Geometry: final body of the model. Coordinates: model frame, mm. A direction names the side the tool comes from. Give positions to 0.01 mm unless a question says otherwise; leave off trailing zeros. Write each loop counter-clockwise with the first axis right and the second up, starting at its lowest first coordinate (ties: lowest second). Pieces come first, ordered by that corner, then holes.
```python
from build123d import *

# Parameters (mm, degrees)
SKETCH1_R           = 31.5
BOSS_EXTRUDE4_DEPTH = 10
SKETCH3_R           = 3
CUT_EXTRUDE2_DEPTH  = 10
SKETCH4_R           = 5
CUT_EXTRUDE3_DEPTH  = 5
SKETCH5_R           = 2.5
BOSS_EXTRUDE5_DEPTH = 13


with BuildPart() as part:
    # Sketch1 → Boss-Extrude4 (new body)
    with BuildSketch(Plane(origin=(0, 0, 0), x_dir=(1, 0, 0), z_dir=(0, 1, 0))):
        with Locations(Location((0, 0, 0), (0, 0, 270))):
            Circle(SKETCH1_R)
    extrude(amount=BOSS_EXTRUDE4_DEPTH)

    # Sketch3 → Cut-Extrude2 (cut)
    with BuildSketch(Plane(origin=(0, 0, 0), x_dir=(1, 0, 0), z_dir=(0, 1, 0))):
        with Locations(Location((0, 25, 0), (0, 0, 270))):
            Circle(SKETCH3_R)
        with Locations(Location((25, 0, 0), (0, 0, 270))):
            Circle(SKETCH3_R)
        with Locations(Location((0, -25, 0), (0, 0, 270))):
            Circle(SKETCH3_R)
        with Locations(Location((-25, 0, 0), (0, 0, 270))):
            Circle(SKETCH3_R)
    extrude(amount=CUT_EXTRUDE2_DEPTH, mode=Mode.SUBTRACT)

    # Sketch4 → Cut-Extrude3 (cut)
    with BuildSketch(Plane(origin=(0, 0, 0), x_dir=(1, 0, 0), z_dir=(0, 1, 0))):
        with Locations(Location((0, 25, 0), (0, 0, 270))):
            Circle(SKETCH4_R)
        with Locations(Location((25, 0, 0), (0, 0, 270))):
            Circle(SKETCH4_R)
        with Locations(Location((0, -25, 0), (0, 0, 270))):
            Circle(SKETCH4_R)
        with Locations(Location((-25, 0, 0), (0, 0, 270))):
            Circle(SKETCH4_R)
    extrude(amount=CUT_EXTRUDE3_DEPTH, mode=Mode.SUBTRACT)

    # Sketch5 → Boss-Extrude5 (add)
    with BuildSketch(Plane(origin=(0, 0, 0), x_dir=(1, 0, 0), z_dir=(0, 1, 0))):
        with BuildLine():
            Line((-40.658639918, -26.516504294), (26.516504294, 40.658639918))
            ThreePointArc((26.516504294, 40.658639918), (40.658639918, 40.658639918), (40.658639918, 26.516504294))
            Line((40.658639918, 26.516504294), (-26.516504294, -40.658639918))
            ThreePointArc((-26.516504294, -40.658639918), (-40.658639918, -40.658639918), (-40.658639918, -26.516504294))
        make_face()
        with Locations(Location((-33.587572106, -33.587572106, 0), (0, 0, 270))):
            Circle(SKETCH5_R, mode=Mode.SUBTRACT)
        with Locations(Location((33.587572106, 33.587572106, 0), (0, 0, 270))):
            Circle(SKETCH5_R, mode=Mode.SUBTRACT)
    extrude(amount=-BOSS_EXTRUDE5_DEPTH)


solid = part.part
```
Item 1: Section A-A, the plane x = 0. Return the cut outline in (y, z).
Found:
outline: (-13, -14.14) - (0, -14.14) - (0, -20) - (5, -20) - (5, -22) - (10, -22) - (10, 22) - (5, 22) - (5, 20) - (0, 20) - (0, 14.14) - (-13, 14.14) - close; (0, -31.5) - (10, -31.5) - (10, -28) - (5, -28) - (5, -30) - (0, -30) - close; (0, 30) - (5, 30) - (5, 28) - (10, 28) - (10, 31.5) - (0, 31.5) - close
Item 2: Section B-B, the plane z = 24. Return the cut outline in (x, y).
Found:
outline: (-38.14, -13) - (-9.86, -13) - (-9.86, 0) - (-4.9, 0) - (-4.9, 5) - (-2.83, 5) - (-2.83, 10) - (-20.4, 10) - (-20.4, 0) - (-38.14, 0) - close; (2.83, 5) - (4.9, 5) - (4.9, 0) - (20.4, 0) - (20.4, 10) - (2.83, 10) - close
Item 3: Reachability of faces 5 (the face through (-29.88, 2.46, -1.08)), 6 (the face through (14, 0, 13)), 7 (the face through (-13, 0, -14)), 8 (the face through (40.501, -6.409, -40.812)), 9 (the face through (31.232, 4.93, -4.101)) from +Z, -Z, +X, -X, +Y, -Y: full face, straight path, thin tool, end or side. Return the list, or none.
Found:
face 5: -Y
face 6: +Z, +X, -Y
face 7: -Z, -X, -Y
face 8: +Y, -Y
face 9: +Y
Item 4: Line query: L1, parallel to X at y = 7.5, z = 0; L2, parallel to X at y = 3, z = 0. Output: solid intervals per line, ascending.
Found:
L1: x = -31.5 to -28, -22 to 22, 28 to 31.5
L2: x = -31.5 to -30, -20 to 20, 30 to 31.5
Item 5: Pin query (flat end, axial travel): pin 1 Ø2 at (x, y) = (-24, -4) entering from -Z; pin 2 Ø16 at (x, z) = (0, -25) entering from -Y; pin 3 Ø8 at (x, z) = (26, 2) entering from -Y; pin 4 Ø4 at (y, z) = (0.5, 20) entering from +X. Return the tip coordinate at first contact, or that it passes through.
Found:
pin 1: stops at z = 8.86
pin 2: stops at y = -13
pin 3: stops at y = 0
pin 4: stops at x = 25.85
Item 6: Section C-C, the plane x = 25. Return the cut outline in (y, z).
Found:
outline: (-13, -39.14) - (0, -39.14) - (0, -19.16) - (10, -19.16) - (10, -3) - (5, -3) - (5, -5) - (0, -5) - (0, -10.86) - (-13, -10.86) - close; (0, 5) - (5, 5) - (5, 3) - (10, 3) - (10, 19.16) - (0, 19.16) - close
Item 7: Section D-D, the plane z = 0. Return the cut outline in (x, y), plus the area to 3 significant figures.
Found:
outline: (-31.5, 0) - (-30, 0) - (-30, 5) - (-28, 5) - (-28, 10) - (-31.5, 10) - close; (-22, 5) - (-20, 5) - (-20, 0) - (-14.14, 0) - (-14.14, -13) - (14.14, -13) - (14.14, 0) - (20, 0) - (20, 5) - (22, 5) - (22, 10) - (-22, 10) - close; (28, 5) - (30, 5) - (30, 0) - (31.5, 0) - (31.5, 10) - (28, 10) - close
area: 838 mm2
Item 8: Pull-direction query (X, two-part tool) for faces 1 (the face through (25.9, 7.46, 2.86)), 2 (the face through (7.54, -6.41, 6.6)), 3 (the face through (29, 0, -29)), 4 (the face through (-28.3, 5, -0.1)); classes: +X half, -X half, draft (parallel to the pull), parting line (faces both ways), or undercut.
Found:
face 1: undercut
face 2: +X half
face 3: draft
face 4: undercut
